```python
from build123d import *

# Parameters (mm, degrees)
SKETCH5_W                      = 301.625
SKETCH5_H                      = 1.5875
BASE_FLANGE1_DEPTH             = 381
SKETCH10_W                     = 11.1125
SKETCH10_H                     = 12.7
BOSS_EXTRUDE1_DEPTH            = 1.5875
EDGE_FLANGE1_STRIP_W           = 12.7
EDGE_FLANGE1_STRIP_H           = 1.5875
EDGE_FLANGE1_STRIP_CUT_DEPTH   = 368.3
EDGE_FLANGE1_STRIP_2_W         = 12.7
EDGE_FLANGE1_STRIP_2_H         = 1.5875
EDGE_FLANGE1_STRIP_CUT_2_DEPTH = 368.3
EDGE_FLANGE1_DEPTH             = 368.3
EDGE_FLANGE1_BEND_DEPTH        = 368.3
CUT_EXTRUDE1_START             = -25.4
CUT_EXTRUDE1_DEPTH             = 342.9
EDGE_FLANGE2_STRIP_W           = 11.43
EDGE_FLANGE2_STRIP_H           = 1.5875
EDGE_FLANGE2_STRIP_CUT_DEPTH   = 25.4
EDGE_FLANGE2_DEPTH             = 25.4
EDGE_FLANGE3_STRIP_W           = 11.43
EDGE_FLANGE3_STRIP_H           = 1.5875
EDGE_FLANGE3_STRIP_CUT_DEPTH   = 25.4
EDGE_FLANGE3_DEPTH             = 25.4
FILLET1_R                      = 8
FILLET2_R                      = 3.175
SKETCH30_W                     = 4
SKETCH30_H                     = 1.5875
CUT_EXTRUDE9_DEPTH             = 4
SKETCH31_W                     = 4
SKETCH31_H                     = 1.5875
CUT_EXTRUDE10_DEPTH            = 4
FILLET4_R                      = 1.5


# Sheet-metal steps are written as plain solids
with BuildPart() as part:
    # Sketch5 → Base-Flange1 (new body)
    with BuildSketch(Plane.XY):
        with Locations((0, -0.79375)):
            Rectangle(SKETCH5_W, SKETCH5_H)
    extrude(amount=BASE_FLANGE1_DEPTH)

    # Sketch10 → Boss-Extrude1 (add)
    with BuildSketch(Plane(origin=(0, 0, 0), x_dir=(1, 0, 0), z_dir=(0, 1, 0))):
        with Locations((-156.36875, -6.35)):
            Rectangle(SKETCH10_W, SKETCH10_H)
        with Locations((156.36875, -6.35)):
            Rectangle(SKETCH10_W, SKETCH10_H)
    extrude(amount=-BOSS_EXTRUDE1_DEPTH)

    # Edge-Flange1 strip (across the edge) → Edge-Flange1 strip cut (cut)
    with BuildSketch(Plane(origin=(150.8125, -1.5875, 12.7), x_dir=(-1, 0, 0), z_dir=(0, 0, 1))):
        with Locations((-1.5875, -0.79375)):
            Rectangle(EDGE_FLANGE1_STRIP_W, EDGE_FLANGE1_STRIP_H)
    extrude(amount=EDGE_FLANGE1_STRIP_CUT_DEPTH, mode=Mode.SUBTRACT)

    # Edge-Flange1 strip 2 (across the edge) → Edge-Flange1 strip cut 2 (cut)
    with BuildSketch(Plane(origin=(-150.8125, -1.5875, 381), x_dir=(1, 0, 0), z_dir=(0, 0, -1))):
        with Locations((-1.5875, -0.79375)):
            Rectangle(EDGE_FLANGE1_STRIP_2_W, EDGE_FLANGE1_STRIP_2_H)
    extrude(amount=EDGE_FLANGE1_STRIP_CUT_2_DEPTH, mode=Mode.SUBTRACT)

    # Edge-Flange1 section (across the edge) → Edge-Flange1 (add)
    with BuildSketch(Plane(origin=(150.8125, -1.5875, 12.7), x_dir=(-1, 0, 0), z_dir=(0, 0, 1))):
        with BuildLine():
            Line((0, 3.175), (0, 14.4125))
            Line((0, 14.4125), (1.5875, 14.4125))
            Line((1.5875, 14.4125), (1.5875, 3.175))
            ThreePointArc((1.5875, 3.175), (2.51743597, 0.92993597), (4.7625, 0))
            Line((4.7625, 0), (4.7625, -1.5875))
            ThreePointArc((4.7625, -1.5875), (1.394903955, -0.192596045), (0, 3.175))
        make_face()
    extrude(amount=EDGE_FLANGE1_DEPTH)

    # Edge-Flange1 section 2 (across the edge) → Edge-Flange1 bend (add)
    with BuildSketch(Plane(origin=(-150.8125, -1.5875, 381), x_dir=(1, 0, 0), z_dir=(0, 0, -1))):
        with BuildLine():
            Line((0, 3.175), (0, 14.4125))
            Line((0, 14.4125), (1.5875, 14.4125))
            Line((1.5875, 14.4125), (1.5875, 3.175))
            ThreePointArc((1.5875, 3.175), (2.51743597, 0.92993597), (4.7625, 0))
            Line((4.7625, 0), (4.7625, -1.5875))
            ThreePointArc((4.7625, -1.5875), (1.394903955, -0.192596045), (0, 3.175))
        make_face()
    extrude(amount=EDGE_FLANGE1_BEND_DEPTH)

    # Sketch20 → Cut-Extrude1 (cut)
    with BuildSketch(Plane.XY.offset(381).offset(CUT_EXTRUDE1_START)):
        with BuildLine():
            Line((-150.8125, -4.7625), (-150.8125, -16))
            Line((-150.8125, -16), (-149.225, -16))
            Line((-149.225, -16), (-149.225, -4.7625))
            ThreePointArc((-149.225, -4.7625), (-148.29506403, -2.51743597), (-146.05, -1.5875))
            Line((-146.05, -1.5875), (-146.05, 0))
            ThreePointArc((-146.05, 0), (-149.417596045, -1.394903955), (-150.8125, -4.7625))
        make_face()
        with BuildLine():
            Line((149.225, -4.7625), (149.225, -16))
            Line((149.225, -16), (150.8125, -16))
            Line((150.8125, -16), (150.8125, -4.7625))
            ThreePointArc((150.8125, -4.7625), (149.417596045, -1.394903955), (146.05, 0))
            Line((146.05, 0), (146.05, -1.5875))
            ThreePointArc((146.05, -1.5875), (148.29506403, -2.51743597), (149.225, -4.7625))
        make_face()
    extrude(amount=-CUT_EXTRUDE1_DEPTH, mode=Mode.SUBTRACT)

    # Edge-Flange2 strip (across the edge) → Edge-Flange2 strip cut (cut)
    with BuildSketch(Plane(origin=(-150.8125, -16, 355.6), x_dir=(0, 1, 0), z_dir=(0, 0, 1))):
        with Locations((-1.5875, -0.79375)):
            Rectangle(EDGE_FLANGE2_STRIP_W, EDGE_FLANGE2_STRIP_H)
    extrude(amount=EDGE_FLANGE2_STRIP_CUT_DEPTH, mode=Mode.SUBTRACT)

    # Edge-Flange2 section (across the edge) → Edge-Flange2 (add)
    with BuildSketch(Plane(origin=(-150.8125, -16, 355.6), x_dir=(0, 1, 0), z_dir=(0, 0, 1))):
        with BuildLine():
            Line((0, 2.54), (0, 11.1125))
            Line((0, 11.1125), (1.5875, 11.1125))
            Line((1.5875, 11.1125), (1.5875, 2.54))
            ThreePointArc((1.5875, 2.54), (2.331448776, 0.743948776), (4.1275, 0))
            Line((4.1275, 0), (4.1275, -1.5875))
            ThreePointArc((4.1275, -1.5875), (1.208916761, -0.378583239), (0, 2.54))
        make_face()
    extrude(amount=EDGE_FLANGE2_DEPTH)

    # Edge-Flange3 strip (across the edge) → Edge-Flange3 strip cut (cut)
    with BuildSketch(Plane(origin=(150.8125, -16, 381), x_dir=(0, 1, 0), z_dir=(0, 0, -1))):
        with Locations((-1.5875, -0.79375)):
            Rectangle(EDGE_FLANGE3_STRIP_W, EDGE_FLANGE3_STRIP_H)
    extrude(amount=EDGE_FLANGE3_STRIP_CUT_DEPTH, mode=Mode.SUBTRACT)

    # Edge-Flange3 section (across the edge) → Edge-Flange3 (add)
    with BuildSketch(Plane(origin=(150.8125, -16, 381), x_dir=(0, 1, 0), z_dir=(0, 0, -1))):
        with BuildLine():
            Line((0, 2.54), (0, 11.1125))
            Line((0, 11.1125), (1.5875, 11.1125))
            Line((1.5875, 11.1125), (1.5875, 2.54))
            ThreePointArc((1.5875, 2.54), (2.331448776, 0.743948776), (4.1275, 0))
            Line((4.1275, 0), (4.1275, -1.5875))
            ThreePointArc((4.1275, -1.5875), (1.208916761, -0.378583239), (0, 2.54))
        make_face()
    extrude(amount=EDGE_FLANGE3_DEPTH)

    # Fillet1
    fillet1_edges = [part.edges().sort_by_distance(p)[0] for p in [
        (-146.05, -0.79375, 12.7),
        (146.05, -0.79375, 12.7),
    ]]
    fillet(fillet1_edges, radius=FILLET1_R)

    # Fillet2
    fillet2_edges = [part.edges().sort_by_distance(p)[0] for p in [
        (-161.925, -0.79375, 12.7),
        (-161.925, -0.79375, 0),
        (-161.925, -15.20625, 355.6),
        (-161.925, -15.20625, 381),
        (161.925, -15.20625, 381),
        (161.925, -15.20625, 355.6),
        (161.925, -0.79375, 0),
        (161.925, -0.79375, 12.7),
    ]]
    fillet(fillet2_edges, radius=FILLET2_R)

    # Sketch30 → Cut-Extrude9 (cut)
    with BuildSketch(Plane.ZY.offset(146.05)):
        with Locations((353.6, -0.79375)):
            Rectangle(SKETCH30_W, SKETCH30_H)
    extrude(amount=-CUT_EXTRUDE9_DEPTH, mode=Mode.SUBTRACT)

    # Sketch31 → Cut-Extrude10 (cut)
    with BuildSketch(Plane(origin=(146.05, 0, 0), x_dir=(0, 0, -1), z_dir=(1, 0, 0))):
        with Locations((-353.6, -0.79375)):
            Rectangle(SKETCH31_W, SKETCH31_H)
    extrude(amount=-CUT_EXTRUDE10_DEPTH, mode=Mode.SUBTRACT)

    # Fillet4
    fillet4_edges = [part.edges().sort_by_distance(p)[0] for p in [
        (-146.05, -0.79375, 351.6),
        (-142.05, -0.79375, 351.6),
        (-142.05, -0.79375, 355.6),
        (146.05, -0.79375, 351.6),
        (142.05, -0.79375, 351.6),
        (142.05, -0.79375, 355.6),
    ]]
    fillet(fillet4_edges, radius=FILLET4_R)


solid = part.part
```
For this review, take the finished solid that the model builds, in its own axes (mm). A direction names the side the tool comes from. Round coordinates to 2 decimals unless told otherwise and drop trailing zeros. Order: outer loops, then holes, each group sorted by start corner. A loop starts at its lowest first (then second) coordinate and runs counter-clockwise, first axis right, second up. Notation, with made-up numbers: (42.5, 27.5) -> (64.5, 27.5) arc R25 cw to (64.5, 40.5) -> close; hole circle Ø8 at (-21.5, 40). An arc over 180 degrees is marked (long way). Use a Markdown table: item, result.
Item 1: Take a section at A-A (y = -8.75). State the section outline as (x, z) points (1 decimal).
Resolved:
| item | result |
|---|---|
| outline | (-150.8, 355.6) -> (-149.2, 355.6) -> (-149.2, 381) -> (-150.8, 381) -> close; (149.2, 355.6) -> (150.8, 355.6) -> (150.8, 381) -> (149.2, 381) -> close |
Item 2: For pin 1 (5 mm diameter, centred on x = 56.5, z = 318, fed in from -Y); pin 2 (6 mm diameter, centred on x = -50.5, z = 154, fed in from +Y); pin 3 (1.7 mm diameter, centred on x = 157.5, y = -1, fed in from +Z); pin 4 (2.5 mm diameter, centred on x = 157.5, z = 373, fed in from +Y), all flat-tipped, find the tip position at first contact; note any pin that passes through.
Resolved:
| item | result |
|---|---|
| pin 1 | stops at y = -1.59 |
| pin 2 | stops at y = 0 |
| pin 3 | stops at z = 12.7 |
| pin 4 | stops at y = -14.41 |
Item 3: For line 1 along Y through (x, z) = (-116, 329), list the stretches that pass through material, from the lowest coordinate up. Write a range as [from, to].
Resolved:
| item | result |
|---|---|
| line 1 | y = [-1.59, 0] |
Item 4: Machinability: for faces 4 (the flat face through (158, -14.412, 368)), 5 (the flat face through (-158, -14.412, 368)), 6 (the cylindrical face through (-148.456, -0.783, 14.981)), 7 (the cylindrical face through (148.331, -0.805, 15.106)), which of the approach directions +Z, -Z, +X, -X, +Y, -Y give a long, thin tool a straight path to every point of the face, cutting with its end or side? Answer none if there is none.
Resolved:
| item | result |
|---|---|
| face 4 | +Z, -Z, +X, +Y |
| face 5 | +Z, -Z, -X, +Y |
| face 6 | -X, +Y, -Y |
| face 7 | +X, +Y, -Y |
Item 5: Take a section at C-C (z = 228). State the section outline as (x, y) points, plus the area to 3 significant figures.
Resolved:
| item | result |
|---|---|
| outline | (-146.05, -1.59) -> (146.05, -1.59) -> (146.05, 0) -> (-146.05, 0) -> close |
| area | 464 mm² |
Item 6: Draft analysis for pull direction Z (two halves, no side actions). For faces 1 (the flat face through (1, -1, 381)), 2 (the flat face through (150.6, -8.6, 355.6)), 3 (the flat face through (-2, 0, 188)), state which applies: +Z half, -Z half, draft (parallel to the pull), parting line (faces both ways), or undercut.
Resolved:
| item | result |
|---|---|
| face 1 | +Z half |
| face 2 | undercut |
| face 3 | draft |
Item 7: Take a section at B-B (x = -24). State the section outline as (y, z) points, plus the area to 3 significant figures.
Resolved:
| item | result |
|---|---|
| outline | (-1.59, 0) -> (0, 0) -> (0, 381) -> (-1.59, 381) -> close |
| area | 605 mm² |
